```python
from build123d import *

# Parameters (mm, degrees)
F0_R     = 32.4993
F1_DEPTH = 26
F2_R     = 3.175
F4_D     = 3.81


with BuildPart() as f1:
    # F0 (on Front) → F1 (new body)
    with BuildSketch(Plane.XZ):
        Circle(F0_R)
    extrude(amount=F1_DEPTH)

    # F2
    f2_edges = [f1.edges().sort_by_distance(p)[0] for p in [
        (-32.4993, -26, 0),
        (-32.4993, 0, 0),
    ]]
    fillet(f2_edges, radius=F2_R)

    # F4 (through all)
    with Locations(Plane.XZ.offset(26)):
        with Locations((0, 0)):
            Hole(F4_D / 2)


solid = f1.part
```
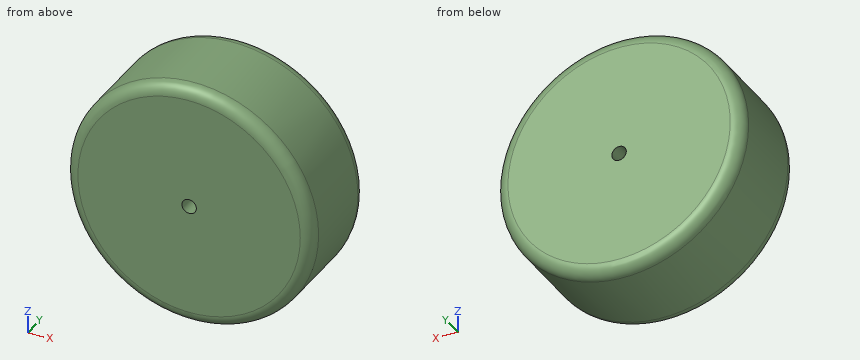
The model under review builds one solid part; all positions refer to its coordinate system, in mm. Give positions to 0.01 mm unless a question says otherwise; leave off trailing zeros. Order: outer loops, then holes, each group sorted by start corner. A loop starts at its lowest first (then second) coordinate and runs counter-clockwise, first axis right, second up. Notation, with made-up numbers: (85.25, 5) - (112.25, 5) arc R26 ccw to (112.25, 34) - close; hole circle Ø4 at (87, 53). An arc over 180 degrees is marked (long way). Use CSV: the item, a comma, the result in double quotes. Start each with the question number.
Q1. We need section C-C, the plane y = -17.25. Write out the cut boundary in (x, z) (3 decimals).
Q2. We need section A-A, the plane z = 0. Write out the cut boundary in (x, y) (3 decimals).
Q3. Clearance check with flat-ended pins moving along their axes: pin 1 Ø5 at (x, y) = (-20, -13.5) entering from -Z; pin 2 Ø5 at (x, y) = (8.5, -18.5) entering from +Z; pin 3 Ø2 at (y, z) = (-17.5, 24) entering from -X. State where each tip first meets the part, or that it passes through.
Q4. To check wall thickness, follow line 1 along Z through (x, y) = (0, -9.25) (3 decimals); line 2 along X through (y, z) = (-6, 14); line 3 along X through (y, z) = (-24.5, -1.5). State the ranges of each line that lie inside material, in increasing order. Write a range as [from, to].
Q5. We need section B-B, the plane x = 0. Write out the cut boundary in (y, z) (3 decimals).
Outcome:
1,outline,"circle Ø64.999 at (0, 0); hole circle Ø3.81 at (0, 0)"
2,outline,"(-32.499, -22.825) arc R3.175 ccw to (-29.324, -26) - (-1.905, -26) - (-1.905, 0) - (-29.324, 0) arc R3.175 ccw to (-32.499, -3.175) - close; (1.905, -26) - (29.324, -26) arc R3.175 ccw to (32.499, -22.825) - (32.499, -3.175) arc R3.175 ccw to (29.324, 0) - (1.905, 0) - close"
3,pin 1,"stops at z = -27.39"
3,pin 2,"stops at z = 31.94"
3,pin 3,"stops at x = -22.96"
4,line 1,"z = [-32.499, -1.905], [1.905, 32.499]"
4,line 2,"x = [-29.33, 29.33]"
4,line 3,"x = [-31.99, -1.17], [1.17, 31.99]"
5,outline,"(-26, -29.324) arc R3.175 ccw to (-22.825, -32.499) - (-3.175, -32.499) arc R3.175 ccw to (0, -29.324) - (0, -1.905) - (-26, -1.905) - close; (-26, 1.905) - (0, 1.905) - (0, 29.324) arc R3.175 ccw to (-3.175, 32.499) - (-22.825, 32.499) arc R3.175 ccw to (-26, 29.324) - close"
